Design review of the part shown in the three views and the two pictorial views. Dimensions are in mm from the part's minimum x, y and z. A direction names the side the tool comes from. Round coordinates to 2 decimals unless told otherwise and drop trailing zeros. Loops run counter-clockwise (first coordinate to the right, second up) from the corner with the lowest first, then second, coordinate; pieces in that order, holes last.
1. Consider section B-B on x = 48. State the section outline as (y, z) points, then the cut area to 3 significant figures.
2. Consider section C-C on y = 27.5. State the section outline as (x, z) points (1 decimal), then the cut area to 3 significant figures.
3. Consider section D-D on z = 13. State the section outline as (x, y) points, then the cut area to 3 significant figures.
4. Tool access review of the marked faces 1, 2 and 3: name each direction out of +Z, -Z, +X, -X, +Y, -Y from which nothing blocks a thin tool from reaching the whole face with its end or side.
5. To check wall thickness, follow line 1 along X through (y, z) = (36, 24) (1 decimal); line 2 along Y through (x, z) = (27, 73); line 3 along X through (y, z) = (8, 5) (1 decimal). State the ranges of each line that lie inside material, in increasing order.
6. Clearance check with flat-ended pins moving along their axes: pin 1 Ø7.5 at (x, y) = (68, 35.5) entering from +Z; pin 2 Ø8 at (x, z) = (33, 12) entering from +Y; pin 3 Ø19.5 at (x, y) = (52, 37) entering from -Z. State where each tip first meets the part, or that it passes through.
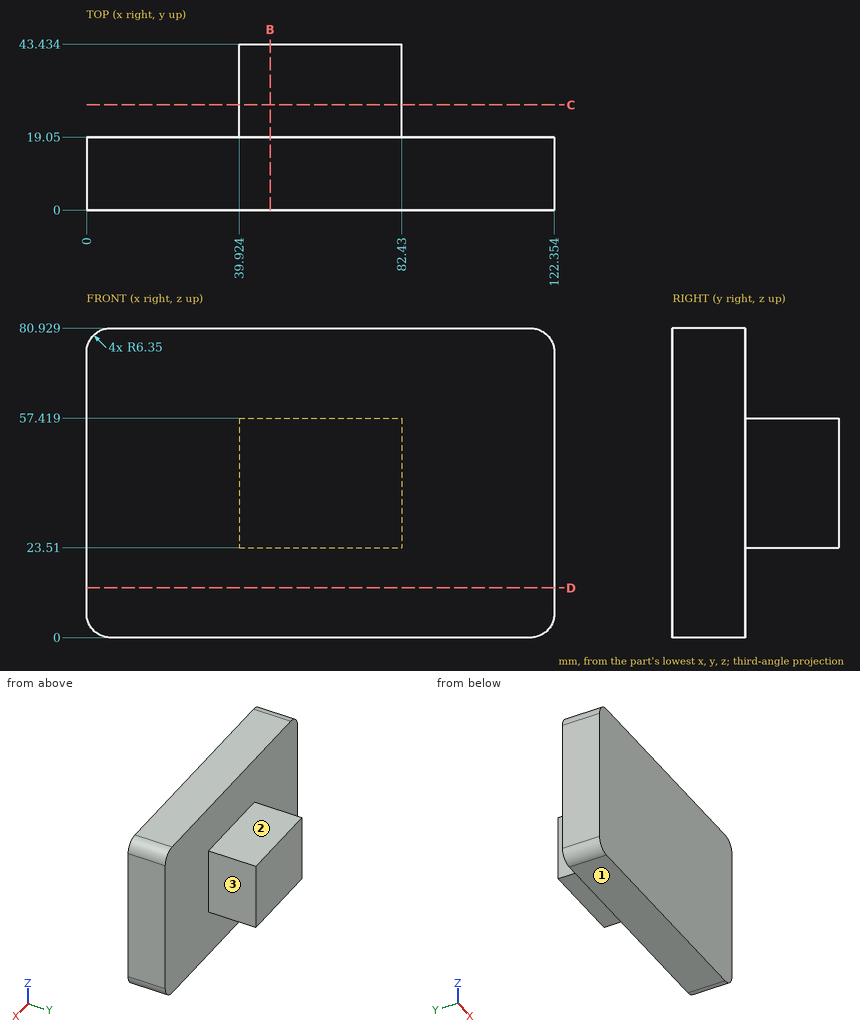
Resolved:
1. outline: (0, 0) - (19.05, 0) - (19.05, 23.51) - (43.43, 23.51) - (43.43, 57.42) - (19.05, 57.42) - (19.05, 80.93) - (0, 80.93) - close
1. area: 2,370 mm2
2. outline: (39.9, 23.5) - (82.4, 23.5) - (82.4, 57.4) - (39.9, 57.4) - close
2. area: 1,440 mm2
3. outline: (0, 0) - (122.35, 0) - (122.35, 19.05) - (0, 19.05) - close
3. area: 2,330 mm2
4. face 1: -Z, +X, -X, +Y, -Y
4. face 2: +Z, +X, -X, +Y
4. face 3: +Z, -Z, +X, +Y
5. line 1: x = 39.9 to 82.4
5. line 2: y = 0 to 19.05
5. line 3: x = 0.1 to 122.2
6. pin 1: stops at z = 57.42
6. pin 2: stops at y = 19.05
6. pin 3: stops at z = 23.51
